```python
from build123d import *

# Parameters (mm, degrees)
SKETCH_2_W          = 90
SKETCH_2_H          = 70
EXTRUDE_1_DEPTH     = 7
EXTRUDE_4_DEPTH     = 7
SKETCH_9_R          = 5.5
EXTRUDE_5_DEPTH     = 79
EXTRUDE_START       = 79
SKETCH_10_R         = 7.5
EXTRUDE_6_DEPTH     = 4
EXTRUDE_7_DEPTH     = 83
CUT_EXTRUDE_1_DEPTH = 10
FILLET_START        = -1
FILLET_1_DEPTH      = 92
FILLET_2_R          = 1
FILLET_3_R          = 1.5
FILLET_4_R          = 1.5
FILLET_9_R          = 1
FILLET_10_R         = 1
FILLET_12_R         = 2


with BuildPart() as part:
    # Sketch 2 → Extrude 1 (new body)
    with BuildSketch(Plane(origin=(0, 0, 0), x_dir=(1, 0, 0), z_dir=(0, 1, 0))):
        with Locations((45, 35)):
            Rectangle(SKETCH_2_W, SKETCH_2_H)
    extrude(amount=-EXTRUDE_1_DEPTH)



with BuildPart() as body_2:
    # Sketch 4 → Extrude 4 (new body)
    with BuildSketch(Plane(origin=(0, 0, 0), x_dir=(0, 0, -1), z_dir=(1, 0, 0))):
        with BuildLine():
            Line((0, 0), (30.669872981, 53.121778265))
            ThreePointArc((30.669872981, 53.121778265), (35, 55.621778265), (39.330127019, 53.121778265))
            Line((39.330127019, 53.121778265), (70, 0))
            Line((70, 0), (0, 0))
        make_face()
    extrude(amount=EXTRUDE_4_DEPTH)

    # Sketch 9 → Extrude 5 (add)
    with BuildSketch(Plane(origin=(7, 0, 0), x_dir=(0, 0, -1), z_dir=(1, 0, 0))):
        with Locations((35, 40)):
            Circle(SKETCH_9_R)
    extrude(amount=EXTRUDE_5_DEPTH)

    # Sketch 10 → Extrude 6 (add)
    with BuildSketch(Plane(origin=(7, 0, 0), x_dir=(0, 0, -1), z_dir=(1, 0, 0)).offset(EXTRUDE_START)):
        with Locations((35, 40)):
            Circle(SKETCH_10_R)
    extrude(amount=EXTRUDE_6_DEPTH)


with BuildPart() as part_1:
    add(part.part)

    add(body_2.part)  # Extrude 7 merges body 2
    # Sketch 11 → Extrude 7 (add)
    with BuildSketch(Plane(origin=(7, 0, 0), x_dir=(0, 0, -1), z_dir=(1, 0, 0))):
        with BuildLine():
            Line((4.089101615, 7.082531755), (0, 0))
            Line((0, 0), (5, 0))
            Line((5, 0), (7.839101615, 4.917468245))
            ThreePointArc((7.839101615, 4.917468245), (7.04663337, 7.875), (4.089101615, 7.082531755))
        make_face()
    extrude(amount=EXTRUDE_7_DEPTH)

    # Sketch 13 → Cut-Extrude 1 (cut)
    with BuildSketch(Plane.XY):
        with BuildLine():
            Line((22.297230248, 5.078430518), (72.297230248, 5.078430518))
            ThreePointArc((72.297230248, 5.078430518), (73.797230248, 3.578430518), (72.297230248, 2.078430518))
            Line((72.297230248, 2.078430518), (22.297230248, 2.078430518))
            ThreePointArc((22.297230248, 2.078430518), (20.797230248, 3.578430518), (22.297230248, 5.078430518))
        make_face()
    extrude(amount=-CUT_EXTRUDE_1_DEPTH, mode=Mode.SUBTRACT)

    # Fillet 1: read off the stored shape, not the designer's step
    # Fillet 1 outline → Fillet 1 (cut)
    with BuildSketch(Plane.YZ.offset(FILLET_START)):
        with BuildLine():
            Line((0, -70), (0.232050808, -69.866025404))
            ThreePointArc((0.232050808, -69.866025404), (-0.009130147, -69.965925826), (-0.267949192, -70))
            Line((-0.267949192, -70), (0, -70))
        make_face()
    extrude(amount=FILLET_1_DEPTH, mode=Mode.SUBTRACT)

    # Fillet 2
    fillet_2_edges = [part_1.edges().sort_by_distance(p)[0] for p in [
        (45, 0, 0),
    ]]
    fillet(fillet_2_edges, radius=FILLET_2_R)

    # Fillet 3
    fillet_3_edges = [part_1.edges().sort_by_distance(p)[0] for p in [
        (90, 40, -27.5),
    ]]
    fillet(fillet_3_edges, radius=FILLET_3_R)

    # Fillet 4
    fillet_4_edges = [part_1.edges().sort_by_distance(p)[0] for p in [
        (86, 40, -27.5),
    ]]
    fillet(fillet_4_edges, radius=FILLET_4_R)

    # Fillet 9
    fillet_9_edges = [part_1.edges().sort_by_distance(p)[0] for p in [
        (90, 2.458734123, -6.419550808),
        (90, 3.657291281, -2.111538106),
        (90, 7.875, -7.04663337),
        (90, -3.633974596, 0),
        (90, -0.009130147, -0.034074174),
    ]]
    fillet(fillet_9_edges, radius=FILLET_9_R)

    # Fillet 10
    # the kernel refuses this fillet: 1 mm, written as the material it takes off along each edge
    with BuildSketch(Plane(origin=(90, 2.232050808, -70), x_dir=(0, 0, 1), z_dir=(0, -1, 0))) as fillet_10_piece_1:
        with BuildLine():
            CenterArc((FILLET_10_R, FILLET_10_R), FILLET_10_R, 180, 90)
            Line((0, FILLET_10_R), (0, 0))
            Line((0, 0), (FILLET_10_R, 0))
        make_face()
    extrude(amount=11.732050808, mode=Mode.SUBTRACT)

    # Fillet 12
    fillet_12_edges = [part_1.edges().sort_by_distance(p)[0] for p in [
        (7, 40, -29.5),
    ]]
    fillet(fillet_12_edges, radius=FILLET_12_R)


solid = part_1.part
```
Check sheet for the modelled part. Datum: model origin and axes. Units: mm. A direction names the side the tool comes from. Coordinates: 2 decimals unless noted, no trailing zeros. Write each loop counter-clockwise with the first axis right and the second up, starting at its lowest first coordinate (ties: lowest second). Pieces come first, ordered by that corner, then holes. Notation, with made-up numbers: M 10,39.25 L 65,39.25 A19 cw 65,49.25 Z; hole C -17,8.5 d6. An arc over 180 degrees is marked long. Use one line per item in the form item = value.
Item 1: Sectioned sample at C-C, the plane y = 40. Record the cut outline in (x, z).
Answer below:
outline = M 0,-46.91 L 7,-46.91 L 7,-42.5 A2 cw 9,-40.5 L 86,-40.5 L 86,-41 A1.5 ccw 87.5,-42.5 L 88.5,-42.5 A1.5 ccw 90,-41 L 90,-29 A1.5 ccw 88.5,-27.5 L 87.5,-27.5 A1.5 ccw 86,-29 L 86,-29.5 L 9,-29.5 A2 cw 7,-27.5 L 7,-23.09 L 0,-23.09 Z
Item 2: Sectioned sample at A-A, the plane x = 40.5. Record the cut outline in (y, z).
Answer below:
outline = M -7,-70 L -0.27,-70 A1 ccw 0,-69.96 L 0,-5 L 2.08,-6.2 L 2.08,-1.2 L 0.23,-0.13 A1 ccw -0.27,0 L -7,0 Z; M 5.08,-7.92 A2.17 ccw 7.08,-4.09 L 5.08,-2.93 Z; C 40,-35 d11
Item 3: Material ranges on L1, parallel to X at y = 7, z = -20; L2, parallel to Y at x = 44, z = -59.5; L3, parallel to Y at x = 49, z = -38, recorded low to high. Write a range as from..to.
Answer below:
L1 = 0..7
L2 = -7..0
L3 = -7..0, 35.39..44.61
Item 4: Release check for a two-part mould opening along X. For faces 1 (the face through (89.699, 3.467, -2.331)), 2 (the face through (44, -4, 0)), 3 (the face through (47, 5.078, -5)), 4 (the face through (86, 35, -38)) record: pulls with the +X half, pulls with the -X half, needs draft (parallel to the pull), parting line crosses it, or undercut.
Answer below:
face_1 = pulls with the +X half
face_2 = needs draft
face_3 = undercut
face_4 = undercut
Item 5: Gauge pin test, flat ends, axial feed: pin 1 Ø8 at (x, y) = (26.5, 41) entering from -Z; pin 2 Ø5.5 at (x, z) = (35.5, -4) entering from +Y; pin 3 Ø10 at (y, z) = (22.5, -32.5) entering from +X. Record the tip position at first contact, or that the pin passes through.
Answer below:
pin_1 = -40.5
pin_2 = 8.17
pin_3 = 7
Item 6: Sectioned sample at D-D, the plane z = -14.5. Record the cut outline in (x, y), and give its area (3 significant figures).
Answer below:
outline = M 0,-7 L 90,-7 L 90,0 L 7,0 L 7,25.11 L 0,25.11 Z
area = 806 mm^2
Item 7: Sectioned sample at B-B, the plane z = -35. Record the cut outline in (x, y).
Answer below:
outline = M 0,-7 L 90,-7 L 90,0 L 7,0 L 7,32.5 A2 cw 9,34.5 L 86,34.5 L 86,34 A1.5 ccw 87.5,32.5 L 88.5,32.5 A1.5 ccw 90,34 L 90,46 A1.5 ccw 88.5,47.5 L 87.5,47.5 A1.5 ccw 86,46 L 86,45.5 L 9,45.5 A2 cw 7,47.5 L 7,55.62 L 0,55.62 Z
Item 8: Set-up check for faces 5 (the face through (89.7, 2.39, -6.05)), 6 (the face through (90, 40, -35)), 7 (the face through (47.43, 7.85, -7.09)), 8 (the face through (46.961, 45.453, -34.284)), 9 (the face through (73.797, 3.611, -4.515)): record each of +Z, -Z, +X, -X, +Y, -Y from which the full face is reachable in a straight line by a thin tool's end or side.
Answer below:
face_5 = -Z, +X
face_6 = +Z, -Z, +X, +Y, -Y
face_7 = +X
face_8 = none
face_9 = +Z, -Z
